```python
from build123d import *

# Parameters (mm, degrees)
F0_W     = 18
F0_H     = 32
F1_DEPTH = 6
F2_R     = 1.5
F3_DEPTH = 5
F5_R     = 9
F6_DEPTH = 11


with BuildPart() as f1:
    # F0 (on Right) → F1 (new body)
    with BuildSketch(Plane.YZ):
        Rectangle(F0_W, F0_H)
    extrude(amount=-F1_DEPTH)

    # F2 (on face) → F3 (join)
    with BuildSketch(Plane.XY.offset(16)):
        with BuildLine():
            Line((-6, 9), (-15, 8))
            ThreePointArc((-15, 8), (-23, 0), (-15, -8))
            Line((-15, -8), (-6, -9))
            Line((-6, -9), (-6, 9))
        make_face()
        with Locations((-15, 0)):
            Circle(F2_R, mode=Mode.SUBTRACT)
    extrude(amount=-F3_DEPTH)

    # F4: F1 across plane


with BuildPart() as f1_1:
    add(f1.part)
    add(f1.part.mirror(Plane.XY))

    # F5 (on face) → F6 (join)
    with BuildSketch(Plane.YZ):
        Circle(F5_R)
        with BuildLine():
            ThreePointArc((1.5, 4.769696), (0, -5), (-1.5, 4.769696))
            Line((-1.5, 4.769696), (-1.5, 5.75))
            Line((-1.5, 5.75), (1.5, 5.75))
            Line((1.5, 5.75), (1.5, 4.769696))
        make_face(mode=Mode.SUBTRACT)
    extrude(amount=F6_DEPTH)


solid = f1_1.part
```
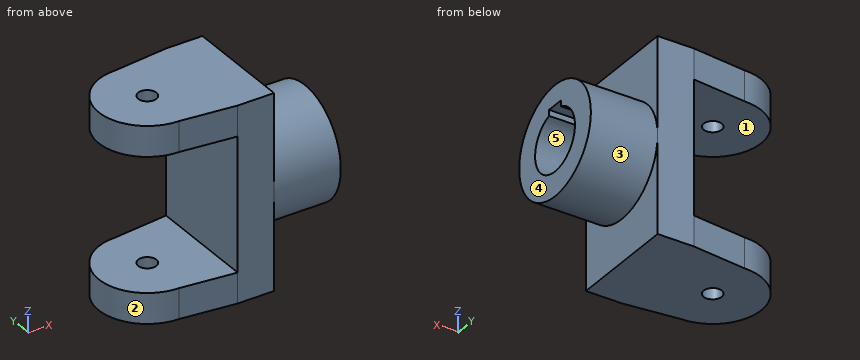
For this review, take the finished solid that the model builds, in its own axes (mm). Face numbers are marked on the shaded views. A direction names the side the tool comes from. Coordinates: 2 decimals unless noted, no trailing zeros. Write each loop counter-clockwise with the first axis right and the second up, starting at its lowest first coordinate (ties: lowest second). Pieces come first, ordered by that corner, then holes. Notation, with made-up numbers: (-17, -35) - (25, -35) arc R29 ccw to (25, -12) - close; hole circle Ø11 at (-20.75, 61). An arc over 180 degrees is marked (long way). Answer in a Markdown table with one row per item. Add a question column.
Q1. We need section A-A, the plane x = -6.5. State the section outline as (y, z) points, and give its area (3 significant figures).
Q2. We need section D-D, the plane x = -15.5. State the section outline as (y, z) points, and give its area (3 significant figures).
Q3. Tool access review of the marked faces 1 and 2: name each direction out of +Z, -Z, +X, -X, +Y, -Y from which nothing blocks a thin tool from reaching the whole face with its end or side.
Q4. We need section C-C, the plane z = 12. State the section outline as (x, y) points, and give its area (3 significant figures).
Q5. Draft analysis for pull direction Z (two halves, no side actions). For the marked faces 3, 4 and 5, state which applies: +Z half, -Z half, draft (parallel to the pull), parting line (faces both ways), or undercut.
Q6. For probe 1 along Z at (x, y) = (-15, -4.25); probe 2 along Y at (x, z) = (1.5, -3); probe 3 along X at (y, z) = (1, -2), list the stretches that pass through material, from the lowest coordinate up.
Q7. For P1, Ø0.5, axis at x = 8, z = 5.5, coming from the -Y side; P2, Ø2.5, axis at x = -15, y = 0, coming from the -Z side; P3, Ø0.5, axis at x = 5, z = 5, coming from the +Y side; P4, Ø4, axis at y = -4.5, z = 8.5, coming from the +X side, all flat-tipped, find the tip position at first contact; note any pin that passes through.
Q8. We need section B-B, the plane y = 0. State the section outline as (x, z) points.
Answer list:
| question | item | result |
|---|---|---|
| 1 | outline | (-8.94, -16) - (8.94, -16) - (8.94, -11) - (-8.94, -11) - close; (-8.94, 11) - (8.94, 11) - (8.94, 16) - (-8.94, 16) - close |
| 1 | area | 179 mm2 |
| 2 | outline | (-7.98, -16) - (-1.41, -16) - (-1.41, -11) - (-7.98, -11) - close; (-7.98, 11) - (-1.41, 11) - (-1.41, 16) - (-7.98, 16) - close; (1.41, -16) - (7.98, -16) - (7.98, -11) - (1.41, -11) - close; (1.41, 11) - (7.98, 11) - (7.98, 16) - (1.41, 16) - close |
| 2 | area | 131 mm2 |
| 3 | face 1 | -X, +Y, -Y |
| 3 | face 2 | +Z, -Z, -X |
| 4 | outline | (-15, -8) - (-6, -9) - (0, -9) - (0, 9) - (-6, 9) - (-15, 8) arc R8 ccw to start; hole circle Ø3 at (-15, 0) |
| 4 | area | 354 mm2 |
| 5 | face 3 | parting line |
| 5 | face 4 | draft |
| 5 | face 5 | undercut |
| 6 | probe 1 | z = -16 to -11, 11 to 16 |
| 6 | probe 2 | y = -8.49 to -4, 4 to 8.49 |
| 6 | probe 3 | x = -6 to 0 |
| 7 | P1 | stops at y = -7.31 |
| 7 | P2 | passes through |
| 7 | P3 | stops at y = 7.64 |
| 7 | P4 | stops at x = 11 |
| 8 | outline | (-23, -16) - (-16.5, -16) - (-16.5, -11) - (-23, -11) - close; (-23, 11) - (-16.5, 11) - (-16.5, 16) - (-23, 16) - close; (-13.5, -16) - (0, -16) - (0, -9) - (11, -9) - (11, -5) - (0, -5) - (0, 5.75) - (11, 5.75) - (11, 9) - (0, 9) - (0, 16) - (-13.5, 16) - (-13.5, 11) - (-6, 11) - (-6, -11) - (-13.5, -11) - close |
